Build history of the part. All positions in model axes, mm. Face numbers are marked on the shaded views. Coordinates: 2 decimals unless noted, no trailing zeros. Loops run counter-clockwise (first coordinate to the right, second up) from the corner with the lowest first, then second, coordinate; pieces in that order, holes last.
Item 1: Mould opens along Z. For the marked faces 1, 2, 3 and 4 say: released by +Z, released by -Z, zero draft, split by the parting line, or undercut.
Item 2: Drill centre lines: line 1 along Y through (x, z) = (5, 0); line 2 along Z through (x, y) = (6.25, -1.5); line 3 along Z through (x, y) = (1.25, 2.75). Where is each one in solid material? Low to high.
Item 3: Cut at A-A (x = 9). List the corners of the cut face in (y, z), and give its area (3 significant figures).
Item 4: Flat gauge pins, fed straight in: pin 1 (1 mm diameter, centred on x = 5.5, y = -1, fed in from -Z); pin 2 (1.5 mm diameter, centred on x = 5, z = 9.5, fed in from -Y); pin 3 (10.5 mm diameter, centred on y = 0, z = 0, fed in from +X); pin 4 (2 mm diameter, centred on x = 4.5, z = 7.5, fed in from -Y). Where does each tip first touch, or does it go through?
Autodesk Inventor part; units mm, degrees
ref_plane "MSC_PT1" through (14.1, 0, 0) normal (1, 0, 0) x (0, 1, 0)
ref_plane "MSC_PT2" through (0, 0, 0) normal (-1, 0, 0) x (0, -1, 0)
ref_plane "MSC_PF1" through (0, 0, 0) normal (1, 0, 0) x (0, 1, 0)
sketch "Sketch1" plane through (0, 0, 0) normal (1, 0, 0) x (0, 1, 0)
  line L0 (10.5, 6.0622) -> (10.5, -6.0622)
  line L1 (10.5, -6.0622) -> (0, -12.1244)
  line L2 (0, -12.1244) -> (-10.5, -6.0622)
  line L3 (-10.5, -6.0622) -> (-10.5, 6.0622)
  line L4 (-10.5, 6.0622) -> (0, 12.1244)
  line L5 (0, 12.1244) -> (10.5, 6.0622)
  circle A0 centre (0, 0) radius 10.5 construction
  dimension "d0" = 21
extrude "Extrusion1" add sketch "Sketch1" along normal blind 14.1
sketch "Sketch2" plane through (14.1, 0, 0) normal (1, 0, 0) x (0, 1, 0)
  line L0 (-10.5, 6.0622) -> (0, 12.1244)
  line L1 (0, -12.1244) -> (-10.5, -6.0622)
  line L2 (-10.5, 6.0622) -> (10.5, -6.0622) construction
  line L3 (-10.5, -6.0622) -> (10.5, 6.0622) construction
  point P0 (0, 0)
hole "Hole1" at (14.1, 0, 0) direction (-1, 0, 0) diameter 13.3762 end through all
chamfer "Chamfer1" distance 1 angle 45 2 edges at (14.1, 0, 6.6881) (0, 0, 6.6881)
sketch "Sketch3" plane through (0, 0, 0) normal (0, 1, 0) x (-1, 0, 0)
  line L0 (-17.0915, 0) -> (3.8489, 0)
  line L1 (-5.7048, 0) -> (0.8574, 0)
  line L2 (-14.1, 0) -> (-14.1, -12.1244)
  line L3 (-14.1, -12.1244) -> (0, -12.1244)
  line L4 (0, -12.1244) -> (0, 0)
  line L5 (-14.1, -6.0622) -> (-14.1, -12.1244)
  line L6 (0, -6.0622) -> (0, -12.1244)
  line L7 (0, -12.1244) -> (-14.1, -12.1244)
  line L8 (-14.1, -10.5) -> (-13.1622, -12.1244)
  line L9 (-14.1, -12.1244) -> (-14.1, -10.5)
  line L10 (-14.1, -12.1244) -> (-13.1622, -12.1244)
  line L11 (0, -10.5) -> (-0.9378, -12.1244)
  line L12 (-0.9378, -12.1244) -> (0, -12.1244)
  line L13 (0, -12.1244) -> (0, -10.5)
  dimension "d32" = 10.5
  dimension "d33" = 30
revolve "Revolution1" cut sketch "Sketch3" angle 360 about axis through (0, 0, 0) along (-1, 0, 0) contours L8 L3 L2 | L4 L3 L11
ref_plane "MSC_PT1" through (14.1, 0, 0) normal (1, 0, 0) x (0, 1, 0)
ref_plane "MSC_PT2" through (0, 0, 0) normal (-1, 0, 0) x (0, -1, 0)
ref_plane "MSC_PF1" through (0, 0, 0) normal (1, 0, 0) x (0, 1, 0)
equation "\"d0\" = Smax"
equation "\"d1\" = Mmax"
equation "\"d10\" = 0.5 * PTC"
equation "\"d32\" = 0.5 * Smax"
equation "\"NND\" = 14"
equation "\"Smax\" = 21"
equation "\"Mmax\" = 14.1"
equation "\"PTC\" = 2"
equation "\"THREADDIA\" = NND"
equation "\"TEMPLATE\" = 1.2345"
properties part number "ANSI B18.2.4.2M - M14x2" material "Steel, Mild"
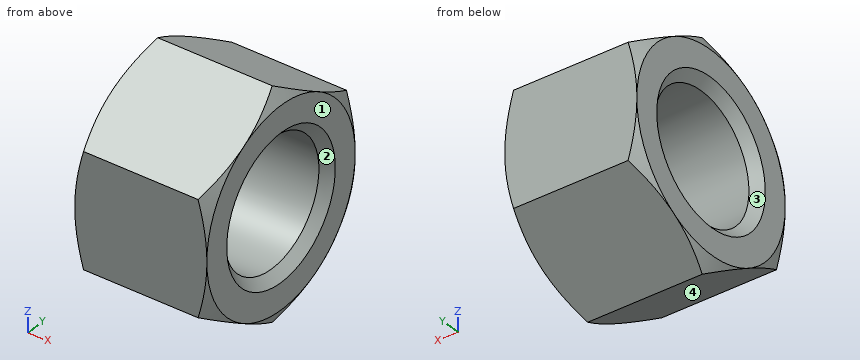
Filled sheet:
1. face 1: zero draft
1. face 2: undercut
1. face 3: undercut
1. face 4: released by -Z
2. line 1: y = -10.5 to -6.69, 6.69 to 10.5
2. line 2: z = -11.26 to -6.52, 6.52 to 11.26
2. line 3: z = -10.54 to -6.1, 6.1 to 10.54
3. outline: (-10.5, -6.06) - (0, -12.12) - (10.5, -6.06) - (10.5, 6.06) - (0, 12.12) - (-10.5, 6.06) - close; hole circle Ø13.38 at (0, 0)
3. area: 241 mm2
4. pin 1: stops at z = -11.84
4. pin 2: stops at y = -5.84
4. pin 3: passes through
4. pin 4: stops at y = -9.74
